Work out the finished part from the listing and answer in its coordinate system (mm). Face numbers are marked on the shaded views. Coordinates: 2 decimals unless noted, no trailing zeros. Order: outer loops, then holes, each group sorted by start corner. A loop starts at its lowest first (then second) coordinate and runs counter-clockwise, first axis right, second up. Notation, with made-up numbers: (1.25, -7) -> (32.25, -7) arc R30 cw to (32.25, 19) -> close; hole circle Ø11 at (15.5, 16). An arc over 180 degrees is marked (long way). Write item = value, one per line. Start each with the question number.
Q1. For a pull along Y with two mould halves and no side action, classify the marked faces 1, 2 and 3 as +Y half, -Y half, draft (parallel to the pull), parting line (faces both ways), or undercut.
Q2. The part is cut by section A-A, the plane z = -2.7. Determine the outline of the cut face in (x, y).
Q3. A flat-ended cylindrical pin translates along its axis: pin 1 (2 mm diameter, centred on x = 0, y = 0, fed in from +Z). Find the tip coordinate at first contact, or state that the pin passes through.
Q4. Straight lines are drawn through the part: L1, parallel to X at y = 0, z = -3.25; L2, parallel to X at y = 1, z = -3.15; L3, parallel to Y at x = -1.15, z = -1.3. For each, find the intervals that lie inside material, in ascending order. Write a range as from..to.
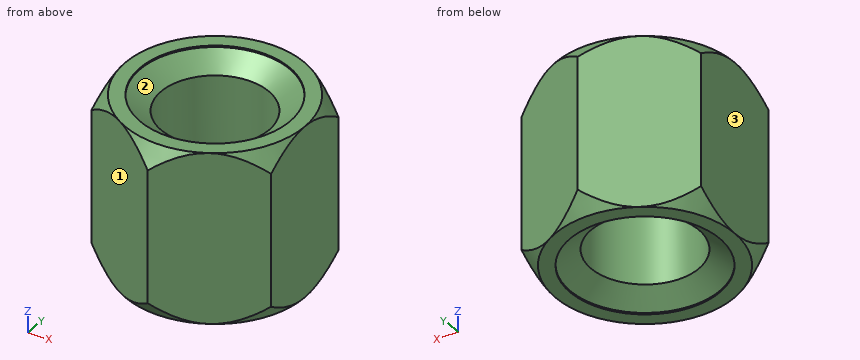
```python
from build123d import *

# Parameters (mm, degrees)
BASENUTSKE_R  = 1.8
BASENUT_DEPTH = 5.7


with BuildPart() as part:
    # BaseNutSke → BaseNut (new body)
    with BuildSketch(Plane.XY):
        Polygon((2.99, 1.726277305), (2.99, -1.726277305), (0, -3.45255461), (-2.99, -1.726277305), (-2.99, 1.726277305), (0, 3.45255461), align=None)
        Circle(BASENUTSKE_R, mode=Mode.SUBTRACT)
    extrude(amount=-BASENUT_DEPTH)

    # Sketch3 → Double-Chamfer (revolve, cut)
    with BuildSketch(Plane(origin=(0, 0, 0), x_dir=(0, 0, -1), z_dir=(1, 0, 0))):
        Polygon((5.7, 2.99), (5.065, 3.45255461), (5.065, 16.15255461), (18.4, 16.15255461), (18.4, 2.99), align=None)
        Polygon((0.635, 16.15255461), (-12.7, 16.15255461), (-12.7, 2.99), (0, 2.99), (0.635, 3.45255461), align=None)
    revolve(axis=Axis((0, 0, 0), (0, 0, -1)), mode=Mode.SUBTRACT)

    # Sketch5 → EndChamfer (revolve, cut)
    with BuildSketch(Plane(origin=(0, 0, 0), x_dir=(0, 0, -1), z_dir=(1, 0, 0))):
        Polygon((5.6502, 2.5), (4.591136098, 0.9875), (5.701, 0.9875), (5.701, 2.5), align=None)
        Polygon((-0.002, 2.5), (0.0488, 2.5), (1.107863902, 0.9875), (-0.002, 0.9875), align=None)
    revolve(axis=Axis((0, 0, -25.037505729), (0, 0, -1)), mode=Mode.SUBTRACT)


solid = part.part
```
Model answer:
q1.face_1 = -Y half
q1.face_2 = undercut
q1.face_3 = draft
q2.outline = (-2.99, -1.73) -> (0, -3.45) -> (2.99, -1.73) -> (2.99, 1.73) -> (0, 3.45) -> (-2.99, 1.73) -> close; hole circle Ø3.6 at (0, 0)
q3.pin_1 = through
q4.L1 = -2.99..-1.8, 1.8..2.99
q4.L2 = -2.99..-1.5, 1.5..2.99
q4.L3 = -2.79..-1.38, 1.38..2.79
